The model under review builds one solid part; all positions refer to its coordinate system, in mm. A direction names the side the tool comes from. Give positions to 0.01 mm unless a question says otherwise; leave off trailing zeros. Loops run counter-clockwise (first coordinate to the right, second up) from the corner with the lowest first, then second, coordinate; pieces in that order, holes last. Notation, with made-up numbers: M -9,74.5 L 43,74.5 A33 ccw 43,111.5 Z; hole C 16,21 d9. An arc over 180 degrees is marked long. Write item = value, one per line. Start each with the question number.
1. For pin 1 (5 mm diameter, centred on x = -4, y = 0, fed in from +Z); pin 2 (3 mm diameter, centred on y = 2.5, z = 17.5, fed in from +X), all flat-tipped, find the tip position at first contact; note any pin that passes through.
2. We need section A-A on y = 0. Give the boundary of the cut face in (x, z).
3. For faces 1 (the face through (0, -3, 33)), 2 (the face through (0, -5, 28)), list the 3-axis set-ups (+Z, -Z, +X, -X, +Y, -Y) from which the entire face can be reached by the end or side of a thin tool; tool diameter is ignored.
4. Wall thickness on line 1 along Z through (x, y) = (2, 0); line 2 along Z through (x, y) = (2, 2.25); line 3 along Y through (x, z) = (4, 5): over which ranges is each line inside the solid? List them lowest first. Write a range as from..to.
5. We need section C-C on z = 5. Give the boundary of the cut face in (x, y).
6. We need section B-B on z = 30.5. Give the boundary of the cut face in (x, y).
from build123d import *

# Parameters (mm, degrees)
SKETCH1_R               = 6
BOSS_EXTRUDE1_DEPTH     = 23
SKETCH2_R               = 2
BOSS_EXTRUDE2_DEPTH     = 10
CHAMFER1_SIZE           = 0.5
CHAMFER2_SIZE           = 0.25
SKETCH3_R               = 1.5
CUT_EXTRUDE1_DEPTH      = 7
CUT_EXTRUDE1_DEPTH_BACK = 7


with BuildPart() as part:
    # Sketch1 → Boss-Extrude1 (new body)
    with BuildSketch(Plane.XY):
        Circle(SKETCH1_R)
    extrude(amount=BOSS_EXTRUDE1_DEPTH)

    # Sketch2 → Boss-Extrude2 (add)
    with BuildSketch(Plane.XY.offset(23)):
        with Locations((0, -3)):
            Circle(SKETCH2_R)
    extrude(amount=BOSS_EXTRUDE2_DEPTH)

    # Chamfer1
    chamfer1_edges = [part.edges().sort_by_distance(p)[0] for p in [
        (-6, 0, 0),
        (-6, 0, 23),
    ]]
    chamfer(chamfer1_edges, length=CHAMFER1_SIZE)

    # Chamfer2
    chamfer2_edges = [part.edges().sort_by_distance(p)[0] for p in [
        (-2, -3, 33),
    ]]
    chamfer(chamfer2_edges, length=CHAMFER2_SIZE)

    # Sketch3 → Cut-Extrude1 (cut, two sides)
    with BuildSketch(Plane(origin=(0, 0, 0), x_dir=(0, 0, -1), z_dir=(1, 0, 0))) as cut_extrude1_sk:
        with Locations((-5, 0)):
            Circle(SKETCH3_R)
    extrude(amount=CUT_EXTRUDE1_DEPTH, mode=Mode.SUBTRACT)
    extrude(cut_extrude1_sk.sketch, amount=-CUT_EXTRUDE1_DEPTH_BACK, mode=Mode.SUBTRACT)


solid = part.part
Final values:
q1.pin_1 = 23
q1.pin_2 = 5.92
q2.outline = M -6,0.5 L -5.5,0 L 5.5,0 L 6,0.5 L 6,3.5 L -6,3.5 Z; M -6,6.5 L 6,6.5 L 6,22.5 L 5.5,23 L -5.5,23 L -6,22.5 Z
q3.face_1 = +Z, +X, -X, +Y, -Y
q3.face_2 = +Z
q4.line_1 = 0..3.5, 6.5..23
q4.line_2 = 0..23
q4.line_3 = -4.47..-1.5, 1.5..4.47
q5.outline = M -5.81,-1.5 A6 ccw 5.81,-1.5 Z; M -5.81,1.5 L 5.81,1.5 A6 ccw Z
q6.outline = C 0,-3 d4
